from build123d import *

# Parameters (mm, degrees)
F0_W     = 76.2
F0_H     = 25.4
F1_DEPTH = 28.575
F2_T     = -2.54
F3_R     = 4.064
F4_DEPTH = 2.54
F5_W     = 12.7
F5_H     = 9.652
F6_DEPTH = 2.54


with BuildPart() as f1:
    # F0 (on Front) → F1 (new body, symmetric)
    with BuildSketch(Plane.XZ):
        with Locations((0.107829, -13.494317)):
            Rectangle(F0_W, F0_H)
    extrude(amount=F1_DEPTH, both=True)

    # F2
    f2_openings = [f1.faces().sort_by_distance(p)[0] for p in [
        (0.107829, 0, -0.794317),
    ]]
    offset(amount=F2_T, openings=f2_openings)

    # F3 (on face) → F4 (cut, through all)
    with BuildSketch(Plane.YZ.offset(38.207829)):
        with Locations((13.913971, -14.016682)):
            Circle(F3_R)
    extrude(amount=-F4_DEPTH, mode=Mode.SUBTRACT)

    # F5 (on face) → F6 (cut, through all)
    with BuildSketch(Plane.YZ.offset(38.207829)):
        with Locations((-16.11085, -12.890838)):
            Rectangle(F5_W, F5_H)
    extrude(amount=-F6_DEPTH, mode=Mode.SUBTRACT)


solid = f1.part
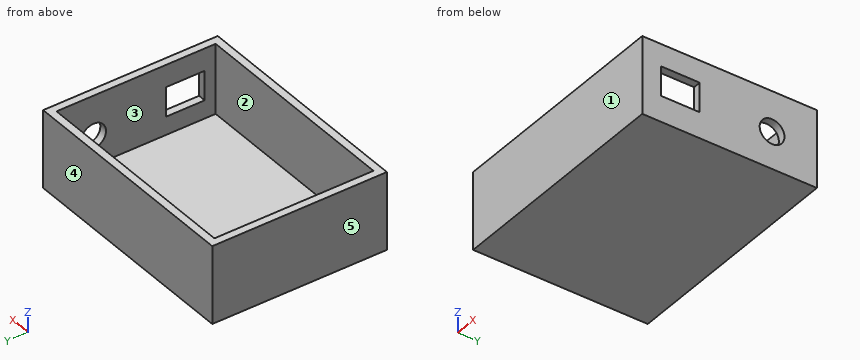
The listing builds one solid part. Answer for the finished solid, in the listing's coordinates (mm). Face numbers are marked on the shaded views. A direction names the side the tool comes from. Round coordinates to 2 decimals unless told otherwise and drop trailing zeros. Write each loop counter-clockwise with the first axis right and the second up, starting at its lowest first coordinate (ties: lowest second). Pieces come first, ordered by that corner, then holes. Notation, with made-up numbers: M 63,63 L 106,63 A13 cw 106,76 Z; hole C 7,-16 d1. An arc over 180 degrees is marked long. Write each question's results on one line, items separated by ' | '. Start each with the question number.
Item 1: Find section D-D on y = -12. Write down the section's boundary in (x, z).
Item 2: Which of the six approach directions +Z, -Z, +X, -X, +Y, -Y give full straight-line access (tool end or side, diameter ignored) to the marked faces 1 and 2?
Item 3: The mould has two halves that part along X. Classify the marked faces 3, 4 and 5: +X half, -X half, draft (parallel to the pull), parting line (faces both ways), or undercut.
Item 4: Given pin 1 Ø6 at (x, y) = (-3, 14.5) entering from +Z, flat-ended and moving along its own axis, determine where the tip first touches the part or whether it passes through.
Item 5: Find section B-B on x = 26. Write down the section's boundary in (y, z) (3 decimals), and give its area (3 significant figures).
Item 6: Straight lines are drawn through the part: probe 1 along X at (y, z) = (-24, -20); probe 2 along Y at (x, z) = (34.5, -20.75) (3 decimals); probe 3 along Z at (x, y) = (25.5, -25). For each, find the intervals that lie inside material, in ascending order.
Item 7: Find section A-A on y = 2.5. Write down the section's boundary in (x, z), and give its area (3 significant figures).
Item 8: Find section C-C on z = -12.5. Write down the section's boundary in (x, y) (3 decimals).
Answer block:
1) outline: M -37.99,-26.19 L 38.21,-26.19 L 38.21,-17.72 L 35.67,-17.72 L 35.67,-23.65 L -35.45,-23.65 L -35.45,-0.79 L -37.99,-0.79 Z; M 35.67,-8.06 L 38.21,-8.06 L 38.21,-0.79 L 35.67,-0.79 Z
2) face 1: +Z, -Z, +X, -X, -Y | face 2: +Z
3) face 3: undercut | face 4: draft | face 5: -X half
4) pin 1: stops at z = -23.65
5) outline: M -28.575,-26.194 L 28.575,-26.194 L 28.575,-0.794 L 26.035,-0.794 L 26.035,-23.654 L -26.035,-23.654 L -26.035,-0.794 L -28.575,-0.794 Z | area: 261 mm²
6) probe 1: x = -37.99 to -35.45, 35.67 to 38.21 | probe 2: y = -28.575 to -26.035, 26.035 to 28.575 | probe 3: z = -26.19 to -23.65
7) outline: M -37.99,-26.19 L 38.21,-26.19 L 38.21,-0.79 L 35.67,-0.79 L 35.67,-23.65 L -35.45,-23.65 L -35.45,-0.79 L -37.99,-0.79 Z | area: 310 mm²
8) outline: M -37.992,-28.575 L 38.208,-28.575 L 38.208,-22.461 L 35.668,-22.461 L 35.668,-26.035 L -35.452,-26.035 L -35.452,26.035 L 35.668,26.035 L 35.668,17.684 L 38.208,17.684 L 38.208,28.575 L -37.992,28.575 Z; M 35.668,-9.761 L 38.208,-9.761 L 38.208,10.144 L 35.668,10.144 Z
